Autodesk Inventor part; units mm, degrees
ref_plane "YZ Plane" through (0, 0, 0) normal (1, 0, 0) x (0, 1, 0)
ref_plane "XZ Plane" through (0, 0, 0) normal (0, 1, 0) x (-1, 0, 0)
ref_plane "XY Plane" through (0, 0, 0) normal (0, 0, 1) x (1, 0, 0)
sketch "Sketch1" plane through (0, 0, 0) normal (0, 0, 1) x (1, 0, 0)
  line L0 (0, 0) -> (52, 0)
  line L1 (52, 0) -> (52, 172)
  line L2 (52, 172) -> (0, 172)
  line L3 (0, 172) -> (0, 0)
  line L4 (0, 0) -> (10, 0)
  line L5 (10, 0) -> (10, 10)
  line L6 (10, 10) -> (0, 10)
  line L7 (0, 10) -> (0, 0)
  circle A0 centre (5, 5) radius 1.7
  line L8 (52, 0) -> (42, 0)
  line L9 (42, 0) -> (42, 10)
  line L10 (42, 10) -> (52, 10)
  line L11 (52, 10) -> (52, 0)
  circle A1 centre (47, 5) radius 1.7
  line L12 (52, 86) -> (47, 86)
  line L13 (0, 172) -> (10, 172)
  line L14 (10, 172) -> (10, 162)
  line L15 (10, 162) -> (0, 162)
  line L16 (0, 162) -> (0, 172)
  circle A2 centre (5, 167) radius 1.7
  line L17 (52, 172) -> (42, 172)
  line L18 (42, 172) -> (42, 162)
  line L19 (42, 162) -> (52, 162)
  line L20 (52, 162) -> (52, 172)
  circle A3 centre (47, 167) radius 1.7
  dimension "d0" = 52
  dimension "d1" = 172
  dimension "d2" = 10
  dimension "d3" = 10
  dimension "d4" = 3.4
extrude "Extrusion1" add sketch "Sketch1" along normal blind 3
sketch "Sketch2" plane through (0, 0, 3) normal (0, 0, 1) x (1, 0, 0)
  circle A0 centre (5, 167) radius 1.7
  circle A1 centre (47, 5) radius 1.7
  line L0 (5, 167) -> (47, 167)
  line L1 (47, 167) -> (47, 5)
  line L2 (47, 5) -> (5, 5)
  line L3 (5, 5) -> (5, 167)
  line L4 (13.3003, 153.806) -> (38.3003, 153.806)
  line L5 (38.3003, 153.806) -> (38.3003, 143.806)
  line L6 (38.3003, 143.806) -> (13.3003, 143.806)
  line L7 (13.3003, 143.806) -> (13.3003, 153.806)
  circle A2 centre (25.8003, 123.7951) radius 10
  line L8 (35.8003, 86) -> (35.8003, 100.6048)
  line L9 (35.8003, 100.6048) -> (26, 100.6048)
  line L10 (35.8003, 100.6048) -> (15.8003, 100.6048)
  line L11 (15.8003, 100.6048) -> (15.8003, 71.4048)
  line L12 (15.8003, 71.4048) -> (35.8003, 71.4048)
  line L13 (35.8003, 71.4048) -> (35.8003, 100.6048)
  line L14 (15.8003, 47.8583) -> (35.8003, 47.8583) construction
  line L15 (15.8003, 52.8601) -> (35.8003, 52.8601)
  line L16 (35.8003, 42.8565) -> (15.8003, 42.8565)
  arc A3 (15.8003, 52.8601) -> (15.8003, 42.8565) centre (15.8003, 47.8583) ccw
  arc A4 (35.8003, 42.8565) -> (35.8003, 52.8601) centre (35.8003, 47.8583) ccw
  line L17 (15.8003, 24.4407) -> (35.8003, 24.4407) construction
  line L18 (15.8003, 19.8936) -> (35.8003, 19.8936)
  line L19 (35.8003, 28.9878) -> (15.8003, 28.9878)
  arc A5 (15.8003, 28.9878) -> (15.8003, 19.8936) centre (15.8003, 24.4407) ccw
  arc A6 (35.8003, 19.8936) -> (35.8003, 28.9878) centre (35.8003, 24.4407) ccw
  point P0 (0, 0)
  point P1 (25.8003, 47.8583)
  point P2 (25.8003, 24.4407)
  dimension "d7" = 25
  dimension "d8" = 10
  dimension "d9" = 20
  dimension "d10" = 29.2
extrude "Extrusion2" cut sketch "Sketch2" against normal blind 3 contours L4 L5 L6 L7 | A2 | L13 L12 L11 L10 L9 L8 | L15 A4 L16 A3 | A5 L19 A6 L18
properties part number "port plugin"
Read the model definition and answer for the solid it produces. Units are mm, in the model's axes. A direction names the side the tool comes from. Coordinates: 2 decimals unless noted, no trailing zeros. Loops run counter-clockwise (first coordinate to the right, second up) from the corner with the lowest first, then second, coordinate; pieces in that order, holes last.
Q1. The part is cut by section C-C on y = 97. Write down the section's boundary in (x, z), and give its area (3 significant figures).
Q2. Consider probe 1 along Y at (x, z) = (47, 1.6); probe 2 along Y at (x, z) = (26, 2.8); probe 3 along Y at (x, z) = (27, 1.7). Determine where each line is inside the solid, lowest interval first.
Q3. The part is cut by section D-D on z = 0.8. Give the number of separate pieces and of enclosed holes in the cut face, and give its area (3 significant figures).
Q4. Each of these flat-tipped pins is pushed along its axis until it touches: pin 1 Ø1.5 at (x, z) = (26.5, 1) entering from -Y; pin 2 Ø2.5 at (x, y) = (47, 5) entering from -Z. Where does it stop, or does it pass through?
Q5. Which of the six approach directions +Z, -Z, +X, -X, +Y, -Y give full straight-line access (tool end or side, diameter ignored) to faces 4 (the face through (0, 87, 1)), 5 (the face through (26, 153.806, 2))?
Q6. The part is cut by section B-B on y = 167. Write down the section's boundary in (x, z).
Q7. The mould has two halves that part along Y. Classify faces 1 (the face through (26, 172, 1)), 2 (the face through (14, 87, 3)), 3 (the face through (26, 71.405, 2)): +Y half, -Y half, draft (parallel to the pull), parting line (faces both ways), or undercut.
Q8. The part is cut by section A-A on x = 47. Write down the section's boundary in (y, z).
Results below:
1. outline: (0, 0) - (15.8, 0) - (15.8, 3) - (0, 3) - close; (35.8, 0) - (52, 0) - (52, 3) - (35.8, 3) - close
1. area: 96.0 mm2
2. probe 1: y = 0 to 3.3, 6.7 to 165.3, 168.7 to 172
2. probe 2: y = 0 to 19.89, 28.99 to 42.86, 52.86 to 71.4, 100.6 to 113.8, 133.79 to 143.81, 153.81 to 172
2. probe 3: y = 0 to 19.89, 28.99 to 42.86, 52.86 to 71.4, 100.6 to 113.87, 133.72 to 143.81, 153.81 to 172
3. separate pieces: 1
3. enclosed holes: 9
3. area: 7,230 mm2
4. pin 1: stops at y = 0
4. pin 2: passes through
5. face 4: +Z, -Z, -X, +Y, -Y
5. face 5: +Z, -Z
6. outline: (0, 0) - (3.3, 0) - (3.3, 3) - (0, 3) - close; (6.7, 0) - (45.3, 0) - (45.3, 3) - (6.7, 3) - close; (48.7, 0) - (52, 0) - (52, 3) - (48.7, 3) - close
7. face 1: +Y half
7. face 2: draft
7. face 3: undercut
8. outline: (0, 0) - (3.3, 0) - (3.3, 3) - (0, 3) - close; (6.7, 0) - (165.3, 0) - (165.3, 3) - (6.7, 3) - close; (168.7, 0) - (172, 0) - (172, 3) - (168.7, 3) - close
